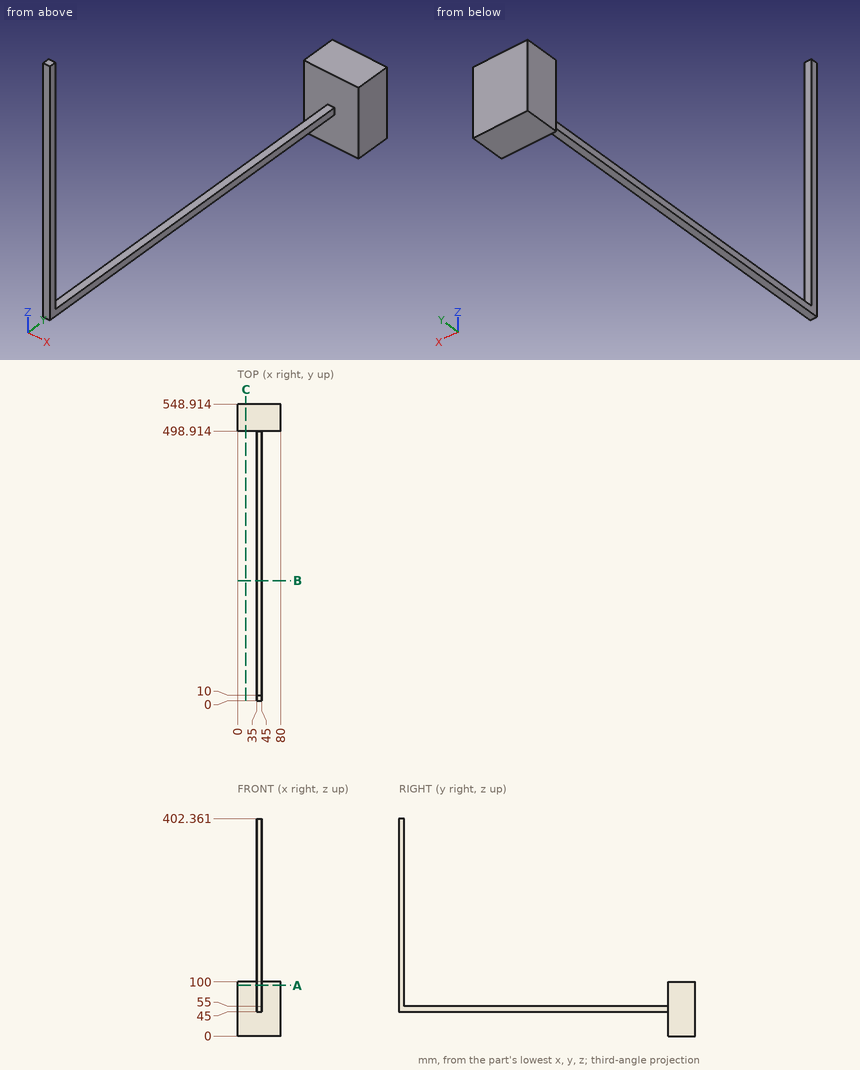
Job drawing, mm, ordinate dimensions from the low corner. One solid piece. Give positions to 0.01 mm unless a question says otherwise; leave off trailing zeros. Order: outer loops, then holes, each group sorted by start corner. A loop starts at its lowest first (then second) coordinate and runs counter-clockwise, first axis right, second up. Notation, with made-up numbers: M -32,64 L -11,64 A28 cw -11,90 Z; hole C 86,78 d5. An arc over 180 degrees is marked long. Return JSON: item names as keys, results as strings.
Q1. Wall check: probe 1 along Y at (x, z) = (36, 232); probe 2 along Z at (x, y) = (36, 121); probe 3 along Y at (x, z) = (69, 55.5). Give the ranges that are in metal, low to high. Write a range as from..to.
Answer list:
{"probe 1": "y = 0..10", "probe 2": "z = 45..55", "probe 3": "y = 498.91..548.91"}
Q2. Band-saw the part on B-B (y = 222). Give the cut face in (x, z).
Answer list:
{"outline": "M 35,45 L 45,45 L 45,55 L 35,55 Z"}
Q3. Band-saw the part on C-C (x = 15.5). Give the cut face in (y, z).
Answer list:
{"outline": "M 498.91,0 L 548.91,0 L 548.91,100 L 498.91,100 Z"}
Q4. Flat gauge pins, fed straight in: pin 1 (8 mm diameter, centred on x = 38, z = 269.5, fed in from +Y); pin 2 (5 mm diameter, centred on x = 38, y = 305.5, fed in from -Z); pin 3 (15 mm diameter, centred on x = 50.5, y = 519, fed in from +Z). Where does each tip first touch, or does it go through?
Answer list:
{"pin 1": "stops at y = 10", "pin 2": "stops at z = 45", "pin 3": "stops at z = 100"}
Q5. Band-saw the part on A-A (z = 93.5). Give the cut face in (x, y), then the cut area to 3 significant figures.
Answer list:
{"outline": "M 0,498.91 L 80,498.91 L 80,548.91 L 0,548.91 Z; M 35,0 L 45,0 L 45,10 L 35,10 Z", "area": "4,100 mm^2"}
